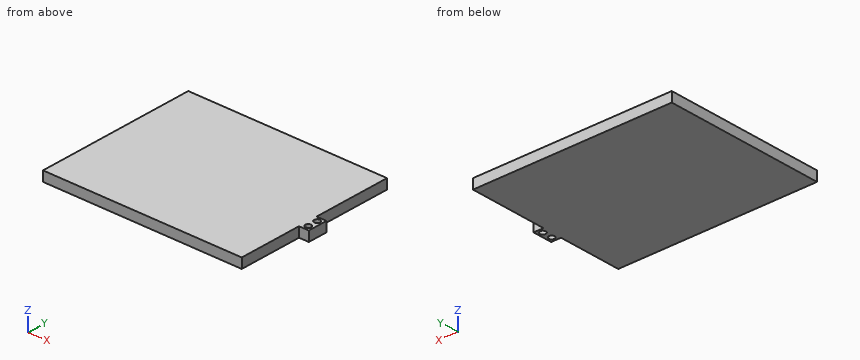
```python
from build123d import *

# Parameters (mm, degrees)
SKETCH2_W           = 256.794
SKETCH2_H           = 196.85
BOSS_EXTRUDE1_DEPTH = 12.7
SKETCH3_W           = 12.7
SKETCH3_H           = 25.4
BOSS_EXTRUDE2_DEPTH = 12.7
SKETCH4_R           = 3.81
CUT_EXTRUDE1_DEPTH  = 12.7
SKETCH5_W           = 256.794
SKETCH5_H           = 12.7
BOSS_EXTRUDE3_DEPTH = 12.7


with BuildPart() as part:
    # Sketch2 → Boss-Extrude1 (new body)
    with BuildSketch(Plane.XY):
        with Locations((5.975438209, -11.247712934)):
            Rectangle(SKETCH2_W, SKETCH2_H)
    extrude(amount=BOSS_EXTRUDE1_DEPTH)

    # Sketch3 → Boss-Extrude2 (add)
    with BuildSketch(Plane(origin=(134.372438209, 0, 0), x_dir=(0, 0, -1), z_dir=(1, 0, 0))):
        with Locations((-6.35, -14.422712934)):
            Rectangle(SKETCH3_W, SKETCH3_H)
    extrude(amount=BOSS_EXTRUDE2_DEPTH)

    # Sketch4 → Cut-Extrude1 (cut)
    with BuildSketch(Plane(origin=(0, 0, 0), x_dir=(-1, 0, 0), z_dir=(0, 0, -1))):
        with Locations((-140.722438209, -8.072712934)):
            Circle(SKETCH4_R)
        with Locations((-140.722438209, -20.772712934)):
            Circle(SKETCH4_R)
    extrude(amount=-CUT_EXTRUDE1_DEPTH, mode=Mode.SUBTRACT)

    # Sketch5 → Boss-Extrude3 (add)
    with BuildSketch(Plane(origin=(0, 87.177287066, 0), x_dir=(1, 0, 0), z_dir=(0, 1, 0))):
        with Locations((5.975438209, -6.35)):
            Rectangle(SKETCH5_W, SKETCH5_H)
    extrude(amount=BOSS_EXTRUDE3_DEPTH)


solid = part.part
```
The listing builds one solid part. Answer for the finished solid, in the listing's coordinates (mm). Round coordinates to 2 decimals unless told otherwise and drop trailing zeros. Loops run counter-clockwise (first coordinate to the right, second up) from the corner with the lowest first, then second, coordinate; pieces in that order, holes last.
Q1. Section A-A, the plane z = 3.75 is taken. Determine the outline of the cut face in (x, y).
Q2. Given pin 1 Ø4 at (y, z) = (51, 7.5) entering from +X; pin 2 Ø4 at (x, z) = (138.5, 6.5) entering from -Y, each flat-ended and moving along its own axis, determine where each tip first touches the part or whether it passes through.
Q3. Section B-B, the plane y = 2.5 is taken. Determine the outline of the cut face in (x, z).
Q4. Find the intervals of material crossed by line 1 (X direction, y = -21, z = 3.75); line 2 (X direction, y = 76.5, z = 10.25); line 3 (X direction, y = -9, z = 4), in increasing order.
Completed:
1. outline: (-122.42, -109.67) - (134.37, -109.67) - (134.37, -27.12) - (147.07, -27.12) - (147.07, -1.72) - (134.37, -1.72) - (134.37, 99.88) - (-122.42, 99.88) - close; hole circle Ø7.62 at (140.72, -20.77); hole circle Ø7.62 at (140.72, -8.07)
2. pin 1: stops at x = 134.37
2. pin 2: stops at y = -27.12
3. outline: (-122.42, 0) - (134.37, 0) - (134.37, 12.7) - (-122.42, 12.7) - close
4. line 1: x = -122.42 to 136.92, 144.53 to 147.07
4. line 2: x = -122.42 to 134.37
4. line 3: x = -122.42 to 137.03, 144.42 to 147.07
